Autodesk Inventor part; units mm, degrees
ref_plane "YZ Plane" through (0, 0, 0) normal (1, 0, 0) x (0, 1, 0)
ref_plane "XZ Plane" through (0, 0, 0) normal (0, 1, 0) x (-1, 0, 0)
ref_plane "XY Plane" through (0, 0, 0) normal (0, 0, 1) x (1, 0, 0)
sketch "Эскиз1" plane through (0, 0, 0) normal (0, 1, 0) x (-1, 0, 0)
  line L0 (0, 0) -> (62.2951, 0) construction
  line L1 (-40, 45) -> (-200, 45)
  line L2 (-200, -45) -> (-40, -45)
  circle A0 centre (-90, 25) radius 2.25
  line L3 (-90, 25) -> (-135, 25) construction
  circle A1 centre (-135, 25) radius 2.25
  circle A2 centre (-90, -25) radius 2.25
  circle A3 centre (-135, -25) radius 2.25
  line L4 (0, 185) -> (20, 185)
  line L5 (50, 155) -> (50, -155)
  line L6 (20, -185) -> (0, -185)
  line L7 (0, 85) -> (0, 185)
  arc A4 (50, 155) -> (20, 185) centre (20, 155) ccw
  arc A5 (20, -185) -> (50, -155) centre (20, -155) ccw
  line L8 (-240, 185) -> (-365, 185)
  line L9 (-590, 185) -> (-590, -185)
  line L10 (-590, -185) -> (-540, -185)
  line L11 (-240, 85) -> (-240, 185)
  arc A6 (-40, 45) -> (0, 85) centre (-40, 85) ccw
  line L12 (0, -185) -> (0, -85)
  arc A7 (0, -85) -> (-40, -45) centre (-40, -85) ccw
  arc A8 (-240, 85) -> (-200, 45) centre (-200, 85) ccw
  line L13 (-240, -185) -> (-240, -85)
  arc A9 (-200, -45) -> (-240, -85) centre (-200, -85) ccw
  line L14 (-365, 185) -> (-365, 100)
  line L15 (-365, 100) -> (-420, 100)
  line L16 (-420, 100) -> (-420, 140)
  line L17 (-420, 140) -> (-485, 140)
  line L18 (-485, 140) -> (-485, 100)
  line L19 (-485, 100) -> (-540, 100)
  line L20 (-540, 100) -> (-540, 185)
  line L21 (-495.3156, 130) -> (-414.5161, 130) construction
  circle A10 centre (-480, 130) radius 2.25
  circle A11 centre (-425, 130) radius 2.25
  line L22 (-452.5, 140) -> (-452.5, 103.3214) construction
  circle A12 centre (-480, 90) radius 2.25
  circle A13 centre (-425, 90) radius 2.25
  line L23 (-540, 185) -> (-590, 185)
  line L24 (-365, 185) -> (-540, 185) construction
  line L25 (-365, -185) -> (-365, -100)
  line L26 (-365, -100) -> (-420, -100)
  line L27 (-420, -100) -> (-420, -140)
  line L28 (-420, -140) -> (-485, -140)
  line L29 (-485, -140) -> (-485, -100)
  line L30 (-485, -100) -> (-540, -100)
  line L31 (-540, -100) -> (-540, -185)
  circle A14 centre (-480, -130) radius 2.25
  circle A15 centre (-425, -130) radius 2.25
  circle A16 centre (-480, -90) radius 2.25
  circle A17 centre (-425, -90) radius 2.25
  line L32 (-540, -185) -> (-365, -185) construction
  line L33 (-365, -185) -> (-240, -185)
  point P0 (50, 185)
  dimension "d10" = 4.5
  dimension "d11" = 45
  dimension "d12" = 25
  dimension "d13" = 90
  dimension "d14" = 50
  dimension "d15" = 370
  dimension "d16" = 30
  dimension "d20" = 350
  dimension "d21" = 40
  dimension "d22" = 40
  dimension "d23" = 90
  dimension "d24" = 40
  dimension "d25" = 40
  dimension "d26" = 240
  dimension "d27" = 50
  dimension "d28" = 55
  dimension "d29" = 45
  dimension "d30" = 65
  dimension "d31" = 55
  dimension "d32" = 85
  dimension "d33" = 4.5
  dimension "d34" = 55
  dimension "d35" = 10
  dimension "d38" = 40
extrude "Выдавливание3" add sketch "Эскиз1" along normal blind 4
fillet "Сопряжение1" radius 10 4 edges at (365, 2, 100) (540, 2, 100) (540, 2, -100) (365, 2, -100)
fillet "Сопряжение2" radius 10 2 edges at (590, 2, -185) (590, 2, 185)
equation "\"d22\" = d21"
equation "\"d24\" = d21"
equation "\"d25\" = d21"
properties part number "00-01-Платформа"
The model under review builds one solid part; all positions refer to its coordinate system, in mm. A direction names the side the tool comes from. Round coordinates to 2 decimals unless told otherwise and drop trailing zeros. Loops run counter-clockwise (first coordinate to the right, second up) from the corner with the lowest first, then second, coordinate; pieces in that order, holes last. Notation, with made-up numbers: M 43.25,-16.75 L 69.25,-16.75 A22 cw 69.25,16.25 Z; hole C -22,-31.75 d7. An arc over 180 degrees is marked long. Answer as CSV lines item,"result".
1. Insertion check: pin 1 Ø12 at (x, z) = (343.5, -145.5) entering from -Y; pin 2 Ø2 at (x, y) = (390.5, 2) entering from -Z; pin 3 Ø1.2 at (x, y) = (145.5, 2.5) entering from +Z; pin 4 Ø1.2 at (x, y) = (454.5, 2) entering from +Z. Each pin has a flat end and moves straight along its axis. Give the tip position at first contact, or say it passes through.
Outcome:
pin 1,"stops at y = 0"
pin 2,"stops at z = -100"
pin 3,"stops at z = 45"
pin 4,"stops at z = 140"
2. We need section D-D (x = 172.5). Give the boundary of the cut face in (y, z), plus the area to 3 significant figures.
Outcome:
outline,"M 0,-45 L 4,-45 L 4,45 L 0,45 Z"
area,"360 mm2"
3. For faces 1 (the face through (227.972, 1.972, 56.406)), 2 (the face through (-41.445, 1.972, -175.979)), 3 (the face through (12.028, 1.972, -56.406)), list the 3-axis set-ups (+Z, -Z, +X, -X, +Y, -Y) from which the entire face can be reached by the end or side of a thin tool; tool diameter is ignored.
Outcome:
face 1,"+Z, +Y, -Y"
face 2,"-Z, -X, +Y, -Y"
face 3,"-Z, +Y, -Y"
4. To check wall thickness, follow L1, parallel to Z at x = 135, y = 2.2; L2, parallel to Z at x = 480, y = 3.05; L3, parallel to X at y = 2, z = 122.5. State the ranges of each line that lie inside material, in increasing order. Write a range as [from, to].
Outcome:
L1,"z = [-45, -27.25], [-22.75, 22.75], [27.25, 45]"
L2,"z = [-140, -132.25], [-127.75, -92.25], [-87.75, 87.75], [92.25, 127.75], [132.25, 140]"
L3,"x = [-50, 0], [240, 365], [420, 485], [540, 590]"
5. We need section C-C (x = 513). Give the boundary of the cut face in (y, z), plus the area to 3 significant figures.
Outcome:
outline,"M 0,-100 L 4,-100 L 4,100 L 0,100 Z"
area,"800 mm2"
6. Draft analysis for pull direction X (two halves, no side actions). For faces 4 (the face through (274, 4, 3)), 5 (the face through (-40.979, 1.972, 176.445)), 6 (the face through (11.406, 1.972, 57.028)), 7 (the face through (228.594, 1.972, -57.028)), state which applies: pulls with the +X half, pulls with the -X half, needs draft (parallel to the pull), parting line crosses it, or undercut.
Outcome:
face 4,"needs draft"
face 5,"pulls with the -X half"
face 6,"undercut"
face 7,"undercut"
7. We need section A-A (z = -69.5). Give the boundary of the cut face in (x, y), plus the area to 4 significant figures.
Outcome:
outline,"M -50,0 L 3.13,0 L 3.13,4 L -50,4 Z; M 236.87,0 L 590,0 L 590,4 L 236.87,4 Z"
area,"1,625 mm2"
8. We need section B-B (y = 2.3). Count the separate pieces of the cut face and the enclosed holes in it, plus the area to 3 significant figures.
Outcome:
separate pieces,"1"
enclosed holes,"12"
area,"146,000 mm2"
